Autodesk Inventor part; units mm, degrees
ref_plane "YZ Plane" through (0, 0, 0) normal (1, 0, 0) x (0, 1, 0)
ref_plane "XZ Plane" through (0, 0, 0) normal (0, 1, 0) x (-1, 0, 0)
ref_plane "XY Plane" through (0, 0, 0) normal (0, 0, 1) x (1, 0, 0)
sketch "草圖1" plane through (0, 0, 0) normal (0, 1, 0) x (-1, 0, 0)
  line L0 (0, 0) -> (-30, 0)
  line L1 (-30, 0) -> (-30, -40)
  line L2 (-30, -40) -> (0, -40)
  line L3 (0, -40) -> (0, 0)
  line L4 (-30, -40) -> (-50, -40)
  line L5 (-50, -40) -> (-50, -20)
  line L6 (-50, -20) -> (-30, -20)
  line L7 (-30, -20) -> (-30, -40)
  dimension "d0" = 40
  dimension "d1" = 20
  dimension "d2" = 20
  dimension "d3" = 30
extrude "擠出1" add sketch "草圖1" along normal blind 20
sketch "草圖2" plane through (0, 0, -40) normal (-1, 0, 0) x (0, 0, 1)
  line L0 (40, 0) -> (40, 20)
  line L1 (40, 20) -> (0, 20)
  line L2 (0, 20) -> (0, 40)
  line L3 (0, 40) -> (40, 40)
  line L4 (40, 40) -> (40, 20)
  dimension "d6" = 20
extrude "擠出2" add sketch "草圖2" against normal blind 10
sketch "草圖3" plane through (50, 0, -40) normal (0, 0, -1) x (-1, 0, 0)
  line L0 (0, 20) -> (40, 20)
  line L1 (50, 40) -> (40, 40)
  line L2 (0, 20) -> (40, 20)
  line L3 (40, 20) -> (40, 40)
  line L4 (40, 40) -> (0, 40)
  line L5 (0, 40) -> (0, 20)
  point P0 (50, 0)
extrude "擠出3" add sketch "草圖3" against normal blind 10
fillet "圓角1" radius 10 3 edges at (50, 40, -35) (5, 40, 0) (30, 10, -20)
properties part number "36"
Model file for the job. Use its own axes, mm. A direction names the side the tool comes from. Coordinates: 2 decimals unless noted, no trailing zeros. Loops run counter-clockwise (first coordinate to the right, second up) from the corner with the lowest first, then second, coordinate; pieces in that order, holes last. Notation, with made-up numbers: (38, 83) -> (51, 83) arc R19 cw to (51, 113) -> close; hole circle Ø10 at (86.5, 64.25). An arc over 180 degrees is marked (long way). Answer as a JSON object with one key per item and string values.
Q1. Cut at C-C (y = 13). List the corners of the cut face in (x, z), and give its area (3 significant figures).
Report:
{"outline": "(0, -40) -> (50, -40) -> (50, -20) -> (40, -20) arc R10 cw to (30, -10) -> (30, 0) -> (0, 0) -> close", "area": "1,620 mm2"}
Q2. Probe probe 1 along Y at (x, z) = (24, -27.5); probe 2 along X at (y, z) = (27, -22.5); probe 3 along Z at (x, y) = (35, 22.5). List the from-to ranges inside material, lowest first.
Report:
{"probe 1": "y = 0 to 20", "probe 2": "x = 0 to 10", "probe 3": "z = -40 to -30"}
Q3. Cut at A-A (y = 29). List the corners of the cut face in (x, z), and give its area (3 significant figures).
Report:
{"outline": "(0, -40) -> (50, -40) -> (50, -30) -> (10, -30) -> (10, 0) -> (0, 0) -> close", "area": "800 mm2"}
Q4. Flat gauge pins, fed straight in: P1, Ø6, axis at x = 20.5, y = 28, coming from the +Z side; P2, Ø9, axis at x = 25.5, z = -11, coming from the +Y side; P3, Ø5, axis at x = 47.5, y = 14.5, coming from the +Z side. Where does each tip first touch, or does it go through?
Report:
{"P1": "stops at z = -30", "P2": "stops at y = 20", "P3": "stops at z = -20"}
Q5. Cut at B-B (z = -28). List the corners of the cut face in (x, y), and give its area (3 significant figures).
Report:
{"outline": "(0, 0) -> (50, 0) -> (50, 20) -> (10, 20) -> (10, 40) -> (0, 40) -> close", "area": "1,200 mm2"}
Q6. 3-axis set-ups, long thin cutter, end or side, ignore diameter. For faces 1 (the cylindrical face through (5.07, 37.15, -3.01)), 2 (the flat face through (30, 10, -5)), 3 (the flat face through (30, 30, -30)): which of +Z, -Z, +X, -X, +Y, -Y reach the whole face in a straight line?
Report:
{"face 1": "+Z, +X, -X, +Y", "face 2": "+Z, +X, +Y, -Y", "face 3": "+Z, +X, +Y"}
